Geometry check sheet. Reference: the model listing, model coordinates, mm. Face numbers are marked on the shaded views. A direction names the side the tool comes from. Give positions to 0.01 mm unless a question says otherwise; leave off trailing zeros. Loops run counter-clockwise (first coordinate to the right, second up) from the corner with the lowest first, then second, coordinate; pieces in that order, holes last. Notation, with made-up numbers: (80.25, 36) - (121.25, 36) arc R26 ccw to (121.25, 66) - close; hole circle Ø8 at (-4.5, -38). An arc over 180 degrees is marked (long way). Use a Markdown table: item, result. Add a question column.
1. Cross-section at B-B on y = 2. Enter the section's corners in (x, z).
2. Draft check along X on the marked faces 1 and 2. Enter one of: pulls with the +X half, pulls with the -X half, needs draft (parallel to the pull), parting line crosses it, or undercut.
3. Depth check by flat-ended pin: P1, Ø6.5, axis at y = 2.5, z = 7.5, coming from the -X side; P2, Ø1, axis at x = -10.5, z = 7, coming from the -Y side; P3, Ø3, axis at x = 0, z = 8, coming from the -Y side. Enter the tip coordinate at first touch or a pass-through.
4. Cross-section at D-D on z = -6.75. Enter the section's corners in (x, y).
5. Material ranges on L1, parallel to Y at x = 9, z = 4.25; L2, parallel to Y at x = -16.5, z = 5; L3, parallel to Z at x = -3, y = -6.75, recorded low to high.
6. Cross-section at A-A on z = 4.5. Enter the section's corners in (x, y), and give its area (3 significant figures).
7. Cross-section at C-C on x = 11.5. Enter the section's corners in (y, z).
8. Set-up check for the marked faces 3, 4 and 5: record each of +Z, -Z, +X, -X, +Y, -Y from which the full face is reachable in a straight line by a thin tool's end or side.
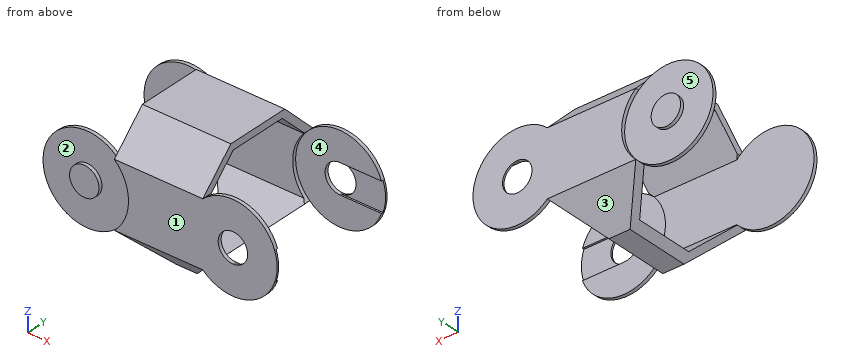
from build123d import *

# Parameters (mm, degrees)
F1_DEPTH  = 7.5
F2_R      = 7.5
F2_R_2    = 2.5
F3_DEPTH  = 11.2
F4_DEPTH  = 11.2
F5_DEPTH  = 10.6
F6_DEPTH  = 10.9
F7_DEPTH  = 10.6
F8_DEPTH  = 11.2
F9_DEPTH  = 10
F12_DEPTH = 22.4


with BuildPart() as f1:
    # F0 (on Right) → F1 (new body, symmetric)
    with BuildSketch(Plane.YZ):
        Polygon((-5, 10), (0, 10), (0, 11.2), (-5.497056, 11.2), (-11.2, 5.497056), (-11.2, -5.497056), (-5.497056, -11.2), (0, -11.2), (0, -10), (-5, -10), (-10, -5), (-10, 5), align=None)
    extrude(amount=F1_DEPTH, both=True)

    # F2 (on Front) → F3 (cut)
    with BuildSketch(Plane.XZ):
        with Locations((-12.602193, 0)):
            Circle(F2_R)
        with Locations((-12.602193, 0)):
            Circle(F2_R_2, mode=Mode.SUBTRACT)
        with BuildLine():
            Line((12.602193, 2.5), (19.673261, 2.5))
            ThreePointArc((19.673261, 2.5), (5.102193, 0), (19.673261, -2.5))
            Line((19.673261, -2.5), (12.602193, -2.5))
            ThreePointArc((12.602193, -2.5), (10.102193, 0), (12.602193, 2.5))
        make_face()
    extrude(amount=F3_DEPTH, mode=Mode.SUBTRACT)

    # F2 (on Front) → F4 (join)
    with BuildSketch(Plane.XZ):
        with BuildLine():
            Line((12.602193, 2.5), (19.673261, 2.5))
            ThreePointArc((19.673261, 2.5), (5.102193, 0), (19.673261, -2.5))
            Line((19.673261, -2.5), (12.602193, -2.5))
            ThreePointArc((12.602193, -2.5), (10.102193, 0), (12.602193, 2.5))
        make_face()
        with BuildLine():
            ThreePointArc((19.673261, -2.5), (19.994182, -1.268265), (20.102193, 0))
            ThreePointArc((20.102193, 0), (19.994182, 1.268265), (19.673261, 2.5))
            Line((19.673261, 2.5), (12.602193, 2.5))
            ThreePointArc((12.602193, 2.5), (14.36996, 1.767767), (15.102193, 0))
            ThreePointArc((15.102193, 0), (14.36996, -1.767767), (12.602193, -2.5))
            Line((12.602193, -2.5), (19.673261, -2.5))
        make_face()
    extrude(amount=F4_DEPTH)

    # F2 (on Front) → F5 (cut)
    with BuildSketch(Plane.XZ):
        with BuildLine():
            Line((12.602193, 2.5), (19.673261, 2.5))
            ThreePointArc((19.673261, 2.5), (5.102193, 0), (19.673261, -2.5))
            Line((19.673261, -2.5), (12.602193, -2.5))
            ThreePointArc((12.602193, -2.5), (10.102193, 0), (12.602193, 2.5))
        make_face()
        with BuildLine():
            ThreePointArc((19.673261, -2.5), (19.994182, -1.268265), (20.102193, 0))
            ThreePointArc((20.102193, 0), (19.994182, 1.268265), (19.673261, 2.5))
            Line((19.673261, 2.5), (12.602193, 2.5))
            ThreePointArc((12.602193, 2.5), (14.36996, 1.767767), (15.102193, 0))
            ThreePointArc((15.102193, 0), (14.36996, -1.767767), (12.602193, -2.5))
            Line((12.602193, -2.5), (19.673261, -2.5))
        make_face()
        with BuildLine():
            ThreePointArc((15.102193, 0), (14.36996, 1.767767), (12.602193, 2.5))
            ThreePointArc((12.602193, 2.5), (10.102193, 0), (12.602193, -2.5))
            ThreePointArc((12.602193, -2.5), (14.36996, -1.767767), (15.102193, 0))
        make_face()
    extrude(amount=F5_DEPTH, mode=Mode.SUBTRACT)

    # F2 (on Front) → F6 (cut)
    with BuildSketch(Plane.XZ):
        with BuildLine():
            ThreePointArc((15.102193, 0), (14.36996, 1.767767), (12.602193, 2.5))
            ThreePointArc((12.602193, 2.5), (10.102193, 0), (12.602193, -2.5))
            ThreePointArc((12.602193, -2.5), (14.36996, -1.767767), (15.102193, 0))
        make_face()
        with BuildLine():
            ThreePointArc((19.673261, -2.5), (19.994182, -1.268265), (20.102193, 0))
            ThreePointArc((20.102193, 0), (19.994182, 1.268265), (19.673261, 2.5))
            Line((19.673261, 2.5), (12.602193, 2.5))
            ThreePointArc((12.602193, 2.5), (14.36996, 1.767767), (15.102193, 0))
            ThreePointArc((15.102193, 0), (14.36996, -1.767767), (12.602193, -2.5))
            Line((12.602193, -2.5), (19.673261, -2.5))
        make_face()
    extrude(amount=F6_DEPTH, mode=Mode.SUBTRACT)

    # F2 (on Front) → F7 (join)
    with BuildSketch(Plane.XZ):
        with Locations((-12.602193, 0)):
            Circle(F2_R)
        with Locations((-12.602193, 0)):
            Circle(F2_R_2, mode=Mode.SUBTRACT)
    extrude(amount=F7_DEPTH)

    # F2 (on Front) → F8 (join)
    with BuildSketch(Plane.XZ):
        with Locations((-12.602193, 0)):
            Circle(F2_R_2)
    extrude(amount=F8_DEPTH)

    # F2 (on Front) → F9 (cut)
    with BuildSketch(Plane.XZ):
        with Locations((-12.602193, 0)):
            Circle(F2_R)
        with Locations((-12.602193, 0)):
            Circle(F2_R_2, mode=Mode.SUBTRACT)
        with Locations((-12.602193, 0)):
            Circle(F2_R_2)
    extrude(amount=F9_DEPTH, mode=Mode.SUBTRACT)

    # F10: F1 across plane


with BuildPart() as f1_1:
    add(f1.part)
    add(f1.part.mirror(Plane.XZ))

    # F11 (on face) → F12 (cut)
    with BuildSketch(Plane.XZ.offset(11.2)):
        Polygon((7.5, -11.2), (7.5, -5.497056), (1.797056, -11.2), align=None)
        Polygon((-1.797056, -11.2), (-7.5, -5.497056), (-7.5, -11.2), align=None)
    extrude(amount=-F12_DEPTH, mode=Mode.SUBTRACT)


solid = f1_1.part
Values found:
| question | item | result |
|---|---|---|
| 1 | outline | (-7.5, 10) - (7.5, 10) - (7.5, 11.2) - (-7.5, 11.2) - close; (-3, -10) - (-1.8, -11.2) - (1.8, -11.2) - (3, -10) - close |
| 2 | face 1 | needs draft |
| 2 | face 2 | undercut |
| 3 | P1 | stops at x = -7.5 |
| 3 | P2 | stops at y = -10.6 |
| 3 | P3 | stops at y = -10.2 |
| 4 | outline | (-15.87, -10.6) - (-9.33, -10.6) - (-9.33, -10) - (-15.87, -10) - close; (-15.87, 10) - (-9.33, 10) - (-9.33, 10.6) - (-15.87, 10.6) - close; (-6.25, -9.95) - (6.25, -9.95) - (6.25, -8.25) - (-6.25, -8.25) - close; (-6.25, 8.25) - (6.25, 8.25) - (6.25, 9.95) - (-6.25, 9.95) - close; (9.33, -11.2) - (15.87, -11.2) - (15.87, -10.6) - (9.33, -10.6) - close; (9.33, 10.6) - (15.87, 10.6) - (15.87, 11.2) - (9.33, 11.2) - close |
| 5 | L1 | y = -11.2 to -10.6, 10.6 to 11.2 |
| 5 | L2 | y = -10.6 to -10, 10 to 10.6 |
| 5 | L3 | z = -9.95 to -8.25, 8.25 to 9.95 |
| 6 | outline | (-18.6, -10.6) - (-6.6, -10.6) - (-6.6, -11.2) - (18.6, -11.2) - (18.6, -10.6) - (6.6, -10.6) - (6.6, -10) - (-18.6, -10) - close; (-18.6, 10) - (6.6, 10) - (6.6, 10.6) - (18.6, 10.6) - (18.6, 11.2) - (-6.6, 11.2) - (-6.6, 10.6) - (-18.6, 10.6) - close |
| 6 | area | 60.5 mm2 |
| 7 | outline | (-11.2, -7.42) - (-10.6, -7.42) - (-10.6, -2.24) - (-11.2, -2.24) - close; (-11.2, 2.24) - (-10.6, 2.24) - (-10.6, 7.42) - (-11.2, 7.42) - close; (10.6, -7.42) - (11.2, -7.42) - (11.2, -2.24) - (10.6, -2.24) - close; (10.6, 2.24) - (11.2, 2.24) - (11.2, 7.42) - (10.6, 7.42) - close |
| 8 | face 3 | -Z, +Y |
| 8 | face 4 | +X |
| 8 | face 5 | +Y |
